Study the drawing (mm; zero at the part's minimum x, y, z) and answer. Coordinates: 2 decimals unless noted, no trailing zeros. Loops run counter-clockwise (first coordinate to the right, second up) from the corner with the lowest first, then second, coordinate; pieces in that order, holes last. Notation, with made-up numbers: (87.25, 60.25) - (96.25, 60.25) arc R18 cw to (96.25, 76.25) - close; hole circle Ø7 at (-4.5, -39.5). An arc over 180 degrees is marked (long way). Write each question's results on one line, items separated by ' | '. Start each with the question number.
(1) Determine the mould class of the marked faces 1, 2, 3 and 4 for opening direction Y: released by +Y, released by -Y, zero draft, split by the parting line, or undercut.
(2) Find section A-A on y = 10. Determine the outline of the cut face in (x, z), then the cut area to 3 significant figures.
(3) Find section B-B on z = 4.9. Determine the outline of the cut face in (x, y).
(4) Find section D-D on y = 18. Determine the outline of the cut face in (x, z), then the cut area to 3 significant figures.
(5) Consider line 1 (X direction, y = 9.75, z = 1.75); line 2 (Y direction, x = 12, z = 6); line 3 (X direction, y = 18.05, z = 4.9). Determine where each line is inside the solid, lowest interval first. Write a range as from..to.
(6) Find section C-C on x = 10. State how many separate pieces and enclosed holes the cut face has, then the cut area to 3 significant figures.
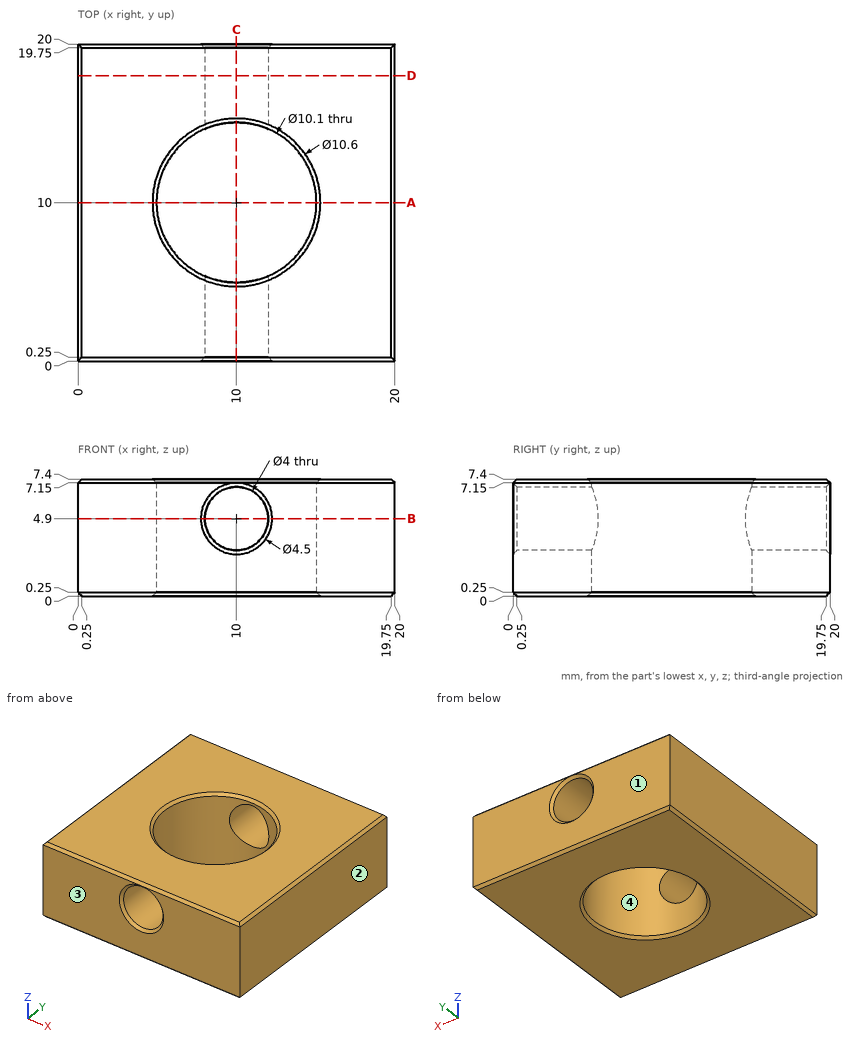
Values:
1) face 1: released by +Y | face 2: zero draft | face 3: released by -Y | face 4: undercut
2) outline: (0, 0.25) - (0.25, 0) - (4.7, 0) - (4.95, 0.25) - (4.95, 7.15) - (4.7, 7.4) - (0.25, 7.4) - (0, 7.15) - close; (15.05, 0.25) - (15.3, 0) - (19.75, 0) - (20, 0.25) - (20, 7.15) - (19.75, 7.4) - (15.3, 7.4) - (15.05, 7.15) - close | area: 73.0 mm²
3) outline: (0, 0) - (7.75, 0) - (8, 0.25) - (8, 5.36) arc R5.05 cw to (8, 14.64) - (8, 19.75) - (7.75, 20) - (0, 20) - close; (12, 0.25) - (12.25, 0) - (20, 0) - (20, 20) - (12.25, 20) - (12, 19.75) - (12, 14.64) arc R5.05 cw to (12, 5.36) - close
4) outline: (0, 0.25) - (0.25, 0) - (19.75, 0) - (20, 0.25) - (20, 7.15) - (19.75, 7.4) - (0.25, 7.4) - (0, 7.15) - close; hole circle Ø4 at (10, 4.9) | area: 135 mm²
5) line 1: x = 0..4.96, 15.04..20 | line 2: y = 0..5.36, 14.64..20 | line 3: x = 0..8, 12..20
6) separate pieces: 4 | enclosed holes: 0 | area: 33.3 mm²
